Design review of the part built by this model. Coordinates are the model's own, in mm. Face numbers are marked on the shaded views. Coordinates: 2 decimals unless noted, no trailing zeros. Answer as a JSON object with one key per item and string values.
Autodesk Inventor part; units mm, degrees
ref_plane "YZ Plane" through (0, 0, 0) normal (1, 0, 0) x (0, 1, 0)
ref_plane "XZ Plane" through (0, 0, 0) normal (0, 1, 0) x (-1, 0, 0)
ref_plane "XY Plane" through (0, 0, 0) normal (0, 0, 1) x (1, 0, 0)
sketch "Sketch1" plane through (0, 0, 0) normal (0, 0, 1) x (1, 0, 0)
  circle A0 centre (0, 0) radius 40.5
  circle A1 centre (0, 0) radius 55.5
  dimension "d0" = 81
  dimension "d1" = 111
extrude "Extrusion1" add sketch "Sketch1" along normal blind 7 contours A0 | A1
sketch "Sketch2" plane through (0, 0, 7) normal (0, 0, 1) x (1, 0, 0)
  circle A0 centre (0, 0) radius 55.5
  circle A1 centre (0, 0) radius 53
  dimension "d4" = 106
extrude "Extrusion2" add sketch "Sketch2" along normal blind 1.5
chamfer "Chamfer1" distance 1.5 angle 15 1 edges at (-53, 0, 7) measured on face at (-39.499, -35.3388, 8)
sketch "Sketch3" plane through (0, 0, 7) normal (0, 0, 1) x (1, 0, 0)
  circle A0 centre (0, 0) radius 5
  dimension "d10" = 10
extrude "Extrusion3" cut sketch "Sketch3" against normal through all
sketch "Sketch4" plane through (0, 0, 7) normal (0, 0, 1) x (1, 0, 0)
  circle A0 centre (0, 0) radius 5
  circle A1 centre (0, 0) radius 39.5
  dimension "d13" = 79
extrude "Extrusion4" add sketch "Sketch4" along normal blind 1.5
sketch "Sketch5" plane through (0, 0, 8.5) normal (0, 0, 1) x (1, 0, 0)
  circle A0 centre (9, 0) radius 1.5
  circle A1 centre (6.364, 6.364) radius 1.5
  circle A2 centre (0, 9) radius 1.5
  circle A3 centre (-6.364, 6.364) radius 1.5
  circle A4 centre (-9, 0) radius 1.5
  circle A5 centre (-6.364, -6.364) radius 1.5
  circle A6 centre (0, -9) radius 1.5
  circle A7 centre (6.364, -6.364) radius 1.5
  point P0 (0, 0)
  dimension "d16" = 3
  dimension "d17" = 9
  dimension "d20" = 360
extrude "Extrusion5" cut sketch "Sketch5" against normal through all
sketch "Sketch7" plane through (0, 0, 0) normal (0, 0, -1) x (-1, 0, 0)
  circle A0 centre (29.5, 0) radius 2
  circle A1 centre (20.8597, 20.8597) radius 2
  circle A2 centre (0, 29.5) radius 2
  circle A3 centre (-20.8597, 20.8597) radius 2
  circle A4 centre (-29.5, 0) radius 2
  circle A5 centre (-20.8597, -20.8597) radius 2
  circle A6 centre (0, -29.5) radius 2
  circle A7 centre (20.8597, -20.8597) radius 2
  point P0 (0, 0)
  dimension "d30" = 4
  dimension "d31" = 29.5
  dimension "d34" = 360
extrude "Extrusion7" cut sketch "Sketch7" against normal through all
sketch "Sketch8" plane through (0, 0, 0) normal (0, 0, -1) x (-1, 0, 0)
  circle A0 centre (0, -29.5) radius 2
  circle A1 centre (-29.5, 0) radius 2
  circle A2 centre (0, 29.5) radius 2
  circle A3 centre (29.5, 0) radius 2
  circle A4 centre (20.8597, 20.8597) radius 2
  circle A5 centre (-20.8597, 20.8597) radius 2
  circle A6 centre (-20.8597, -20.8597) radius 2
  circle A7 centre (20.8597, -20.8597) radius 2
  circle A8 centre (0, -9) radius 1.5
  circle A9 centre (9, 0) radius 1.5
  circle A10 centre (0, 9) radius 1.5
  circle A11 centre (-9, 0) radius 1.5
  circle A12 centre (-6.364, 6.364) radius 1.5
  circle A13 centre (6.364, 6.364) radius 1.5
  circle A14 centre (6.364, -6.364) radius 1.5
  circle A15 centre (-6.364, -6.364) radius 1.5
  circle A16 centre (0, 0) radius 5
  circle A17 centre (0, 0) radius 55.5
extrude "Extrusion8" add sketch "Sketch8" along normal blind 10
sketch "Sketch9" plane through (0, 0, 8.5) normal (0, 0, 1) x (1, 0, 0)
  line L0 (-4.3301, 29.5) -> (-2.1651, 33.25)
  line L1 (-2.1651, 33.25) -> (2.1651, 33.25)
  line L2 (2.1651, 33.25) -> (4.3301, 29.5)
  line L3 (4.3301, 29.5) -> (2.1651, 25.75)
  line L4 (2.1651, 25.75) -> (-2.1651, 25.75)
  line L5 (-2.1651, 25.75) -> (-4.3301, 29.5)
  line L6 (-23.9215, 17.7978) -> (-25.0422, 21.9804)
  line L7 (-25.0422, 21.9804) -> (-21.9804, 25.0422)
  line L8 (-21.9804, 25.0422) -> (-17.7978, 23.9215)
  line L9 (-17.7978, 23.9215) -> (-16.6771, 19.7389)
  line L10 (-16.6771, 19.7389) -> (-19.7389, 16.6771)
  line L11 (-19.7389, 16.6771) -> (-23.9215, 17.7978)
  line L12 (-29.5, -4.3301) -> (-33.25, -2.1651)
  line L13 (-33.25, -2.1651) -> (-33.25, 2.1651)
  line L14 (-33.25, 2.1651) -> (-29.5, 4.3301)
  line L15 (-29.5, 4.3301) -> (-25.75, 2.1651)
  line L16 (-25.75, 2.1651) -> (-25.75, -2.1651)
  line L17 (-25.75, -2.1651) -> (-29.5, -4.3301)
  line L18 (-17.7978, -23.9215) -> (-21.9804, -25.0422)
  line L19 (-21.9804, -25.0422) -> (-25.0422, -21.9804)
  line L20 (-25.0422, -21.9804) -> (-23.9215, -17.7978)
  line L21 (-23.9215, -17.7978) -> (-19.7389, -16.6771)
  line L22 (-19.7389, -16.6771) -> (-16.6771, -19.7389)
  line L23 (-16.6771, -19.7389) -> (-17.7978, -23.9215)
  line L24 (4.3301, -29.5) -> (2.1651, -33.25)
  line L25 (2.1651, -33.25) -> (-2.1651, -33.25)
  line L26 (-2.1651, -33.25) -> (-4.3301, -29.5)
  line L27 (-4.3301, -29.5) -> (-2.1651, -25.75)
  line L28 (-2.1651, -25.75) -> (2.1651, -25.75)
  line L29 (2.1651, -25.75) -> (4.3301, -29.5)
  line L30 (23.9215, -17.7978) -> (25.0422, -21.9804)
  line L31 (25.0422, -21.9804) -> (21.9804, -25.0422)
  line L32 (21.9804, -25.0422) -> (17.7978, -23.9215)
  line L33 (17.7978, -23.9215) -> (16.6771, -19.7389)
  line L34 (16.6771, -19.7389) -> (19.7389, -16.6771)
  line L35 (19.7389, -16.6771) -> (23.9215, -17.7978)
  line L36 (29.5, 4.3301) -> (33.25, 2.1651)
  line L37 (33.25, 2.1651) -> (33.25, -2.1651)
  line L38 (33.25, -2.1651) -> (29.5, -4.3301)
  line L39 (29.5, -4.3301) -> (25.75, -2.1651)
  line L40 (25.75, -2.1651) -> (25.75, 2.1651)
  line L41 (25.75, 2.1651) -> (29.5, 4.3301)
  line L42 (17.7978, 23.9215) -> (21.9804, 25.0422)
  line L43 (21.9804, 25.0422) -> (25.0422, 21.9804)
  line L44 (25.0422, 21.9804) -> (23.9215, 17.7978)
  line L45 (23.9215, 17.7978) -> (19.7389, 16.6771)
  line L46 (19.7389, 16.6771) -> (16.6771, 19.7389)
  line L47 (16.6771, 19.7389) -> (17.7978, 23.9215)
  circle A0 centre (0, 29.5) radius 2
  circle A1 centre (0, 0) radius 5
  point P0 (-20.8597, 20.8597)
  point P1 (-29.5, 0)
  point P2 (-20.8597, -20.8597)
  point P3 (0, -29.5)
  point P4 (20.8597, -20.8597)
  point P5 (29.5, 0)
  point P6 (20.8597, 20.8597)
  dimension "d40" = 7.5
  dimension "d43" = 360
extrude "Extrusion9" cut sketch "Sketch9" against normal blind 5 contours L0 L1 L2 L3 L4 L5 | L6 L7 L8 L9 L10 L11 | L12 L13 L14 L15 L16 L17 | L18 L19 L20 L21 L22 L23 | L24 L25 L26 L27 L28 L29 | L30 L31 L32 L33 L34 L35 | L36 L37 L38 L39 L40 L41 | L42 L43 L44 L45 L46 L47 | A0
properties part number "CS03" material "ABS Plastic"
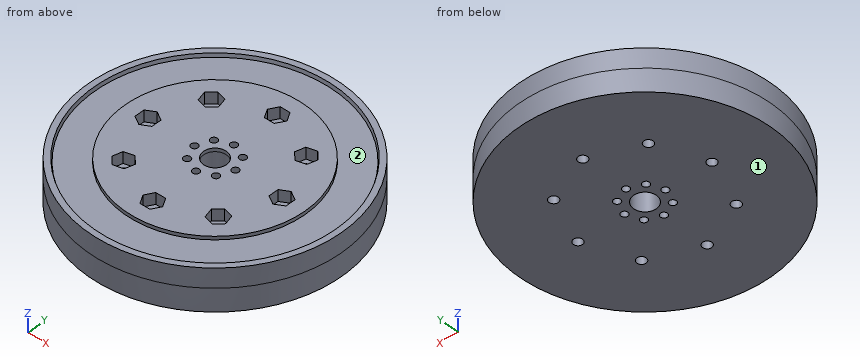
1) Clearance check with flat-ended pins moving along their axes: pin 1 Ø6.5 at (x, y) = (0, 29.5) entering from +Z; pin 2 Ø1 at (x, z) = (31, -2) entering from +Y; pin 3 Ø2.5 at (x, y) = (-20.86, 20.86) entering from +Z; pin 4 Ø3 at (x, z) = (-4, -3) entering from +Y. State where each tip first meets the part, or that it passes through.
Completed:
{"pin 1": "z = 3.5", "pin 2": "y = 46.37", "pin 3": "through", "pin 4": "y = 55.44"}
2) Wall thickness on probe 1 along Y at (x, z) = (0, -5.5); probe 2 along X at (y, z) = (21.5, 4.5); probe 3 along Z at (x, y) = (-42, 23): over which ranges is each line inside the solid? List them lowest first.
Completed:
{"probe 1": "-55.5 to -31.5, -27.5 to -10.5, -7.5 to -5, 5 to 7.5, 10.5 to 27.5, 31.5 to 55.5", "probe 2": "-51.17 to -24.91, -17.15 to 17.15, 24.91 to 51.17", "probe 3": "-10 to 7"}
3) Add section A-A, the plane z = -3. Count the separate pieces of the cut face and the enclosed holes in it, and give its area (3 significant figures).
Completed:
{"separate pieces": "1", "enclosed holes": "17", "area": "9,440 mm²"}
4) The part is to be moulded in two halves that separate along X. For the marked faces 1 and 2, say which applies: pulls with the +X half, pulls with the -X half, needs draft (parallel to the pull), parting line crosses it, or undercut.
Completed:
{"face 1": "needs draft", "face 2": "undercut"}
